from build123d import *

# Parameters (mm, degrees)
F0_W     = 152.4
F0_H     = 152.4
F1_DEPTH = 12.7
F2_R     = 5.08


with BuildPart() as f1:
    # F0 (on Front) → F1 (new body)
    with BuildSketch(Plane.XZ):
        Rectangle(F0_W, F0_H)
    extrude(amount=F1_DEPTH)

    # F2
    f2_edges = [f1.edges().sort_by_distance(p)[0] for p in [
        (76.2, -12.7, 0),
        (0, -12.7, 76.2),
        (-76.2, 0, 0),
        (0, -12.7, -76.2),
        (-76.2, -12.7, 0),
        (0, 0, -76.2),
        (76.2, 0, 0),
        (0, 0, 76.2),
    ]]
    fillet(f2_edges, radius=F2_R)


solid = f1.part
Part model, mm, in its own coordinate system. Give positions to 0.01 mm unless a question says otherwise; leave off trailing zeros. Write each loop counter-clockwise with the first axis right and the second up, starting at its lowest first coordinate (ties: lowest second). Pieces come first, ordered by that corner, then holes.
1) Cut at A-A on y = -10. Write the cut outline in (x, z).
Resolved:
outline: (-75.61, -75.61) - (75.61, -75.61) - (75.61, 75.61) - (-75.61, 75.61) - close
2) Pin check, flat tips, straight feed: pin 1 (2 mm diameter, centred on y = -4, z = -33.5, fed in from +X); pin 2 (4 mm diameter, centred on x = 3.5, y = -10, fed in from +Z). Stop position of each tip, or through.
Resolved:
pin 1: stops at x = 76.2
pin 2: stops at z = 76.19
3) Probe L1, parallel to Z at x = 13, y = -7.75; L2, parallel to Z at x = -35, y = -1.5. List the from-to ranges inside material, lowest first.
Resolved:
L1: z = -76.2 to 76.2
L2: z = -74.72 to 74.72
